Source: CAD feature listing. Evaluate the final solid. Frame: model axes, mm. A direction names the side the tool comes from. Give positions to 0.01 mm unless a question says otherwise; leave off trailing zeros. Write each loop counter-clockwise with the first axis right and the second up, starting at its lowest first coordinate (ties: lowest second). Pieces come first, ordered by that corner, then holes. Notation, with made-up numbers: (-38.75, 84.25) -> (-23.75, 84.25) arc R10 ccw to (-23.75, 94.25) -> close; hole circle Ø2 at (13, -5). An arc over 180 degrees is marked (long way). Answer as a JSON object with one key per item and string values. Group by question number.
Item 1: First-contact query: pin 1 Ø12 at (x, z) = (-5.5, 2.5) entering from -Y; pin 2 Ø6 at (x, y) = (-12.5, 13.5) entering from -Z; pin 3 Ø5.5 at (x, z) = (-12.7, -19.05) entering from -Y; pin 4 Ø4 at (y, z) = (3, -7) entering from -X. Flat tips, straight axial feed; report the tip coordinate or a pass-through.
Item 2: Access query for faces 4 (the face through (-13.97, 9, 3)), 5 (the face through (5, 1, -12.7)), 6 (the face through (-2.1, 14.4, -10.7)), 7 (the face through (-3.668, 5.385, 0.051)), 8 (the face through (-4, 8.334, 4)). Directions: +Z, -Z, +X, -X, +Y, -Y. A direction counts if a zero-diameter tool reaches every point of the face in a straight line with its end or side. Return the directions, or none.
Item 3: Section query A-A on y = 1. Return the cut outline in (x, z), plus the area to 3 significant figures.
Item 4: Section query C-C on x = -12.7. Give the number of separate pieces and of enclosed holes in the cut face, plus the area to 3 significant figures.
Item 5: Pull-direction query (Y, two-part tool) for faces 1 (the face through (-2, 12.875, -7)), 2 (the face through (-4, 7.541, 4)), 3 (the face through (-19.05, 4, -19)); classes: pulls with the +Y half, pulls with the -Y half, needs draft (parallel to the pull), parting line crosses it, or undercut.
Item 6: Ray query, probe 1 along Z at (x, y) = (12.7, 3.75); probe 2 along Z at (x, y) = (-3.81, 11); probe 3 along Z at (x, y) = (-15, 1). Return the intervals inside material, ascending. Write a range as from..to.
Item 7: Section query B-B on z = -19.05. Return the cut outline in (x, y), plus the area to 3 significant figures.
from build123d import *

# Parameters (mm, degrees)
SKETCH1_W                                        = 38.1
SKETCH1_H                                        = 50.8
EXTRUDE1_DEPTH                                   = 15.875
CBORE_FOR_1_4_SOCKET_HEAD_CAP_SCREW1_D           = 6.7564
CBORE_FOR_1_4_SOCKET_HEAD_CAP_SCREW1_CBORE_D     = 11.1125
CBORE_FOR_1_4_SOCKET_HEAD_CAP_SCREW1_CBORE_DEPTH = 6.35
SKETCH3_W                                        = 5.08
SKETCH3_H                                        = 25.4
SKETCH3_W_2                                      = 12.7
CUT_EXTRUDE2_DEPTH                               = 36.497579143
SKETCH5_W                                        = 20.32
SKETCH5_H                                        = 25.4
CUT_EXTRUDE4_DEPTH                               = 1.5875
F_1_4_20_TAPPED_HOLE1_D                          = 5.1054
SKETCH11_W                                       = 19.05
SKETCH11_H                                       = 0.79375
CUT_EXTRUDE5_DEPTH                               = 49.464271634
ADVANCEDHOLE1_START                              = 12.875
ADVANCEDHOLE1_OUTLINE_R                          = 3.25
ADVANCEDHOLE1_DEPTH                              = 3
ADVANCEDHOLE1_START_2                            = 1.5875
ADVANCEDHOLE1_2_OUTLINE_R                        = 1.25
ADVANCEDHOLE1_2_DEPTH                            = 11.2875
ADVANCEDHOLE1_START_3                            = 8.334375
ADVANCEDHOLE1_3_OUTLINE_R                        = 1.55
ADVANCEDHOLE1_3_OUTLINE_R_2                      = 1.25
ADVANCEDHOLE1_3_DEPTH                            = 4.540625


# Read off the part's stored shape, not the designer's step: AdvancedHole1
with BuildPart() as part:
    # Sketch1 → Extrude1 (new body)
    with BuildSketch(Plane(origin=(0, 0, 0), x_dir=(1, 0, 0), z_dir=(0, 1, 0))):
        Rectangle(SKETCH1_W, SKETCH1_H)
    extrude(amount=EXTRUDE1_DEPTH)

    # CBORE for 1/4 Socket Head Cap Screw1 (through all)
    with Locations(Plane(origin=(0, 15.875, 0), x_dir=(-1, 0, 0), z_dir=(0, 1, 0))):
        with Locations((12.7, -19.05), (-12.7, -19.05), (-12.7, 19.05), (12.7, 19.05)):
            CounterBoreHole(CBORE_FOR_1_4_SOCKET_HEAD_CAP_SCREW1_D / 2, CBORE_FOR_1_4_SOCKET_HEAD_CAP_SCREW1_CBORE_D / 2, CBORE_FOR_1_4_SOCKET_HEAD_CAP_SCREW1_CBORE_DEPTH)

    # Sketch3 → Cut-Extrude2 (cut, through all)
    with BuildSketch(Plane(origin=(0, 15.875, 0), x_dir=(-1, 0, 0), z_dir=(0, 1, 0))):
        with Locations((16.51, 0)):
            Rectangle(SKETCH3_W, SKETCH3_H)
        with Locations((-12.7, 0)):
            Rectangle(SKETCH3_W_2, SKETCH3_H)
    extrude(amount=-CUT_EXTRUDE2_DEPTH, mode=Mode.SUBTRACT)

    # Sketch5 → Cut-Extrude4 (cut)
    with BuildSketch(Plane.XZ):
        with Locations((-3.81, 0)):
            Rectangle(SKETCH5_W, SKETCH5_H)
    extrude(amount=-CUT_EXTRUDE4_DEPTH, mode=Mode.SUBTRACT)

    # 1/4-20 Tapped Hole1 (through all)
    with Locations(Plane.ZY.offset(13.97)):
        with Locations((0, 7.9375)):
            Hole(F_1_4_20_TAPPED_HOLE1_D / 2)

    # Sketch11 → Cut-Extrude5 (cut, through all)
    with BuildSketch(Plane(origin=(19.05, 0, 0), x_dir=(0, 0, -1), z_dir=(1, 0, 0))):
        Polygon((25.4, 7.540625), (25.4, 15.875), (12.7, 15.875), (12.7, 8.334375), (12.7, 7.540625), align=None)
        with Locations((3.175, 7.9375)):
            Rectangle(SKETCH11_W, SKETCH11_H)
    extrude(amount=-CUT_EXTRUDE5_DEPTH, mode=Mode.SUBTRACT)

    # AdvancedHole1 outline → AdvancedHole1 (cut)
    with BuildSketch(Plane(origin=(0, 0, 0), x_dir=(1, 0, 0), z_dir=(0, 1, 0)).offset(ADVANCEDHOLE1_START)):
        with Locations((-3.81, 7.9375)):
            Circle(ADVANCEDHOLE1_OUTLINE_R)
    extrude(amount=ADVANCEDHOLE1_DEPTH, mode=Mode.SUBTRACT)

    # AdvancedHole1 2 outline → AdvancedHole1 2 (cut)
    with BuildSketch(Plane(origin=(0, 0, 0), x_dir=(1, 0, 0), z_dir=(0, 1, 0)).offset(ADVANCEDHOLE1_START_2)):
        with Locations((-3.81, 7.9375)):
            Circle(ADVANCEDHOLE1_2_OUTLINE_R)
    extrude(amount=ADVANCEDHOLE1_2_DEPTH, mode=Mode.SUBTRACT)

    # AdvancedHole1 3 outline → AdvancedHole1 3 (cut)
    with BuildSketch(Plane(origin=(0, 0, 0), x_dir=(1, 0, 0), z_dir=(0, 1, 0)).offset(ADVANCEDHOLE1_START_3)):
        with Locations((-3.81, 7.9375)):
            Circle(ADVANCEDHOLE1_3_OUTLINE_R)
        with Locations((-3.81, 7.9375)):
            Circle(ADVANCEDHOLE1_3_OUTLINE_R_2, mode=Mode.SUBTRACT)
    extrude(amount=ADVANCEDHOLE1_3_DEPTH, mode=Mode.SUBTRACT)


solid = part.part
Worked answers:
{
 "1": {"pin 1": "y = 1.59", "pin 2": "z = -12.7", "pin 3": "through", "pin 4": "x = -13.97"},
 "2": {"face 4": "-X, +Y, -Y", "face 5": "-Y", "face 6": "+Y", "face 7": "+X, -X", "face 8": "-Z, +X, -X"},
 "3": {"outline": "(-19.05, -25.4) -> (19.05, -25.4) -> (19.05, -12.7) -> (-19.05, -12.7) -> close; (-19.05, 12.7) -> (19.05, 12.7) -> (19.05, 25.4) -> (-19.05, 25.4) -> close; hole circle Ø6.76 at (-12.7, -19.05); hole circle Ø6.76 at (-12.7, 19.05); hole circle Ø6.76 at (12.7, -19.05); hole circle Ø6.76 at (12.7, 19.05)", "area": "824 mm^2"},
 "4": {"separate pieces": "3", "enclosed holes": "0", "area": "443 mm^2"},
 "5": {"face 1": "pulls with the +Y half", "face 2": "undercut", "face 3": "needs draft"},
 "6": {"probe 1": "-25.4..-22.43, -15.67..-12.7, 12.7..15.67, 22.43..25.4", "probe 2": "-12.7..-9.49, -6.39..25.4", "probe 3": "-25.4..-21.52, -16.58..-12.7, 12.7..16.58, 21.52..25.4"},
 "7": {"outline": "(-19.05, 0) -> (-16.08, 0) -> (-16.08, 7.54) -> (-19.05, 7.54) -> close; (-9.32, 0) -> (9.32, 0) -> (9.32, 7.54) -> (-9.32, 7.54) -> close; (16.08, 0) -> (19.05, 0) -> (19.05, 7.54) -> (16.08, 7.54) -> close", "area": "185 mm^2"}
}
